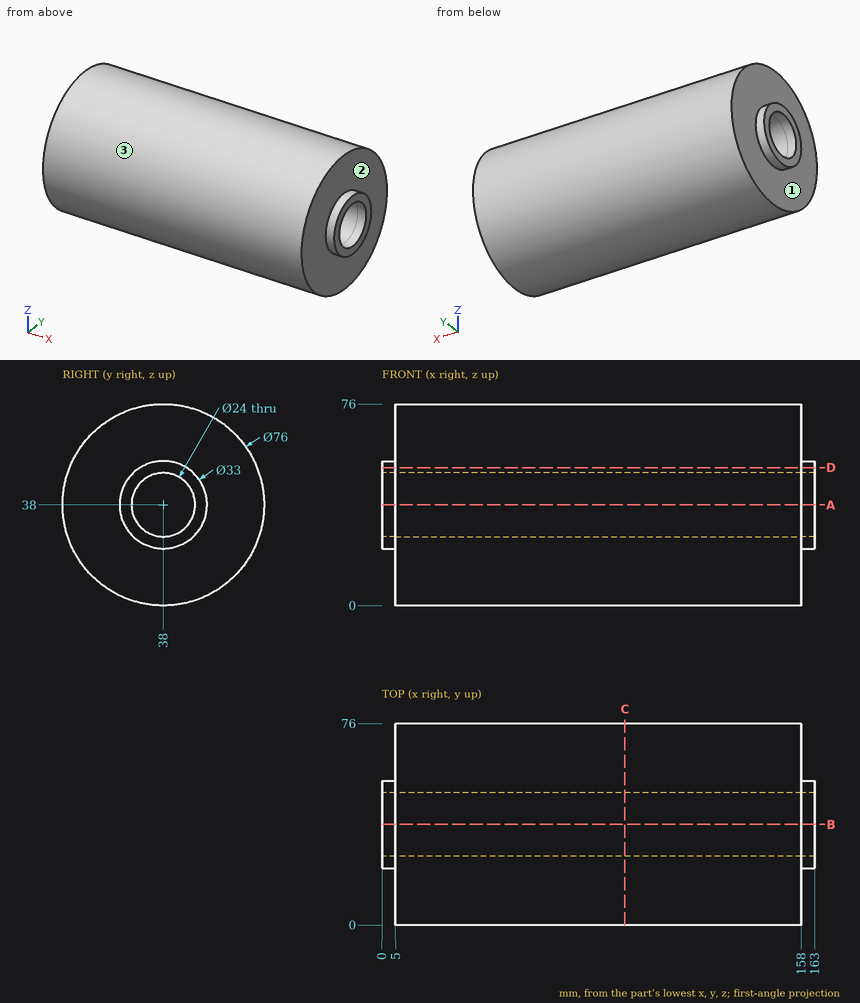
Here's the drawing with two shaded views (mm, measured from the low corner). I have some questions. A direction names the side the tool comes from. Coordinates: 2 decimals unless noted, no trailing zeros. Write each loop counter-clockwise with the first axis right and the second up, starting at its lowest first coordinate (ties: lowest second). Pieces come first, ordered by that corner, then holes.
Item 1: I want a section at C-C on x = 91.5. Write out the boundary of the cut face in (y, z), and give its area (3 significant figures).
Item 2: If I drill on line 1 (Y direction, x = 46.5, z = 38); line 2 (Y direction, x = 161.2, z = 38); line 3 (X direction, y = 50, z = 10), over which ranges is the centre line in solid material (lowest first)?
Item 3: I want a section at D-D on z = 52. Write out the boundary of the cut face in (x, y), and give its area (3 significant figures).
Item 4: I want a section at A-A on z = 38. Write out the boundary of the cut face in (x, y), and give its area (3 significant figures).
Item 5: On a 3-axis mill with a long thin cutter (end or side, diameter ignored), from which of +Z, -Z, +X, -X, +Y, -Y can I reach the whole of each face in a straight line? I mean the marked faces 1, 2 and 3. Say none if no direction works.
Item 6: Will these pins go through, and if not, where does the flat tip stop? pin 1 (4 mm diameter, centred on x = 47.5, y = 44, fed in from -Z); pin 2 (10 mm diameter, centred on x = 111.5, y = 9, fed in from -Z); pin 3 (1.5 mm diameter, centred on x = 56, y = 38.5, fed in from +Z); pin 4 (6 mm diameter, centred on x = 80.5, y = 21.5, fed in from -Z).
Findings below:
1. outline: circle Ø76 at (38, 38); hole circle Ø24 at (38, 38)
1. area: 4,080 mm2
2. line 1: y = 0 to 26, 50 to 76
2. line 2: y = 21.5 to 26, 50 to 54.5
2. line 3: x = 5 to 158
3. outline: (0, 29.27) - (5, 29.27) - (5, 2.67) - (158, 2.67) - (158, 29.27) - (163, 29.27) - (163, 46.73) - (158, 46.73) - (158, 73.33) - (5, 73.33) - (5, 46.73) - (0, 46.73) - close
3. area: 11,000 mm2
4. outline: (0, 21.5) - (5, 21.5) - (5, 0) - (158, 0) - (158, 21.5) - (163, 21.5) - (163, 26) - (0, 26) - close; (0, 50) - (163, 50) - (163, 54.5) - (158, 54.5) - (158, 76) - (5, 76) - (5, 54.5) - (0, 54.5) - close
4. area: 8,050 mm2
5. face 1: -X
5. face 2: +X
5. face 3: +X, -X
6. pin 1: stops at z = 0.21
6. pin 2: stops at z = 8.54
6. pin 3: stops at z = 76
6. pin 4: stops at z = 2.48
